from build123d import *

# Parameters (mm, degrees)
F0_W     = 40
F0_H     = 22.2
F0_R     = 2.125
F0_R_2   = 7.825
F1_DEPTH = 5
F2_R     = 11.1
F2_R_2   = 7.825
F3_DEPTH = 19.5
F4_R     = 11.1
F4_R_2   = 4.75
F5_DEPTH = 5
F6_R     = 11.09999
F7_R     = 2.5


# Not quite as in the source:
# - a fillet or chamfer is up to 0.001 mm smaller than in the source, because OpenCascade refuses the exact size


with BuildPart() as f1:
    # F0 (on Top) → F1 (new body)
    with BuildSketch(Plane.XY):
        Rectangle(F0_W, F0_H)
        with Locations((-15, 0)):
            Circle(F0_R, mode=Mode.SUBTRACT)
        Circle(F0_R_2, mode=Mode.SUBTRACT)
        with Locations((15, 0)):
            Circle(F0_R, mode=Mode.SUBTRACT)
    extrude(amount=F1_DEPTH)

    # F2 (on face) → F3 (join)
    with BuildSketch(Plane.XY.offset(5)):
        Circle(F2_R)
        Circle(F2_R_2, mode=Mode.SUBTRACT)
    extrude(amount=F3_DEPTH)

    # F4 (on face) → F5 (join)
    with BuildSketch(Plane.XY.offset(24.5)):
        Circle(F4_R)
        Circle(F4_R_2, mode=Mode.SUBTRACT)
    extrude(amount=F5_DEPTH)

    # F6 (radius 11.1 in the source; OpenCascade refuses exactly that, so slightly less here)
    f6_edges = [f1.edges().sort_by_distance(p)[0] for p in [
        (-20, 11.1, 2.5),
        (-20, -11.1, 2.5),
        (20, -11.1, 2.5),
        (20, 11.1, 2.5),
    ]]
    fillet(f6_edges, radius=F6_R)

    # F7
    f7_edges = [f1.edges().sort_by_distance(p)[0] for p in [
        (-11.1, 0, 29.5),
    ]]
    fillet(f7_edges, radius=F7_R)


solid = f1.part
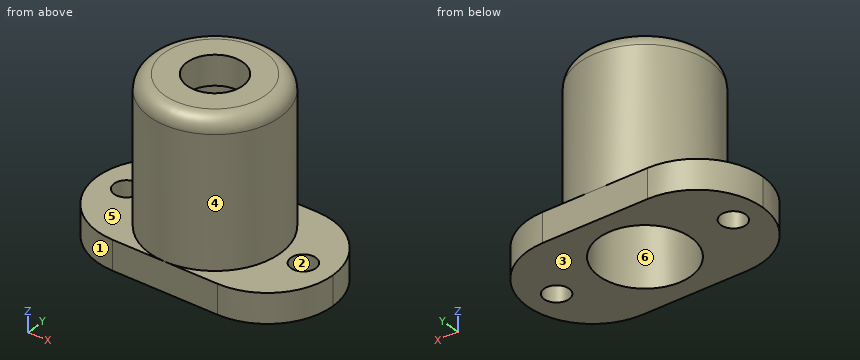
For this review, take the finished solid that the model builds, in its own axes (mm). Face numbers are marked on the shaded views. A direction names the side the tool comes from. Give positions to 0.01 mm unless a question says otherwise; leave off trailing zeros. Loops run counter-clockwise (first coordinate to the right, second up) from the corner with the lowest first, then second, coordinate; pieces in that order, holes last. Notation, with made-up numbers: (87.25, -23.5) -> (100.25, -23.5) arc R12 ccw to (100.25, -9.5) -> close; hole circle Ø2 at (67.25, 62). An arc over 180 degrees is marked (long way). One line per question, with ' | ' between items.
1) We need section B-B (y = 1.5). Give the number of separate pieces and of enclosed holes in the cut face, plus the area to 3 significant figures.
Resolved:
separate pieces: 4 | enclosed holes: 0 | area: 284 mm2
2) Insertion check: pin 1 Ø2 at (y, z) = (4.5, 3) entering from -X; pin 2 Ø4.5 at (x, y) = (-3.5, 1.5) entering from -Z; pin 3 Ø12 at (y, z) = (6, 10.5) entering from +X; pin 4 Ø1.5 at (x, y) = (-10.5, -3) entering from -Z. Each pin has a flat end and moves straight along its axis. Give the tip position at first contact, or say it passes through.
Resolved:
pin 1: stops at x = -19.43 | pin 2: stops at z = 24.5 | pin 3: stops at x = 19.4 | pin 4: stops at z = 0
3) To check wall thickness, follow probe 1 along Y at (x, z) = (0, 16.5) (3 decimals); probe 2 along X at (y, z) = (-0.5, 9.5); probe 3 along Z at (x, y) = (12, 3.5). State the ranges of each line that lie inside material, in increasing order.
Resolved:
probe 1: y = -11.1 to -7.825, 7.825 to 11.1 | probe 2: x = -11.09 to -7.81, 7.81 to 11.09 | probe 3: z = 0 to 5
4) We need section A-A (x = -15). Write out the cut boundary in (y, z) (3 decimals), plus the area to 3 significant figures.
Resolved:
outline: (-9.274, 0) -> (-2.125, 0) -> (-2.125, 5) -> (-9.274, 5) -> close; (2.125, 0) -> (9.274, 0) -> (9.274, 5) -> (2.125, 5) -> close | area: 71.5 mm2
5) We need section C-C (z = 5.5). Write out the cut boundary in (x, y) (3 decimals), plus the area to 3 significant figures.
Resolved:
outline: circle Ø22.2 at (0, 0); hole circle Ø15.65 at (0, 0) | area: 195 mm2
6) The part is to be moulded in two halves that separate along Y. For the marked faces 1, 2 and 3, say which applies: +Y half, -Y half, draft (parallel to the pull), parting line (faces both ways), or undercut.
Resolved:
face 1: -Y half | face 2: undercut | face 3: draft
7) For the marked faces 4, 5 and 6, list the 3-axis set-ups (+Z, -Z, +X, -X, +Y, -Y) from which the entire face can be reached by the end or side of a thin tool; tool diameter is ignored.
Resolved:
face 4: +Z | face 5: +Z, -X | face 6: -Z
